Work out the finished part from the listing and answer in its coordinate system (mm). Coordinates: 2 decimals unless noted, no trailing zeros. Order: outer loops, then holes, each group sorted by start corner. A loop starts at its lowest first (then second) coordinate and runs counter-clockwise, first axis right, second up. Notation, with made-up numbers: M 5,84.5 L 33,84.5 A14 cw 33,98.5 Z; hole C 19,79.25 d8. An arc over 180 degrees is marked long. Use a Markdown table: item, result. Add a question column.
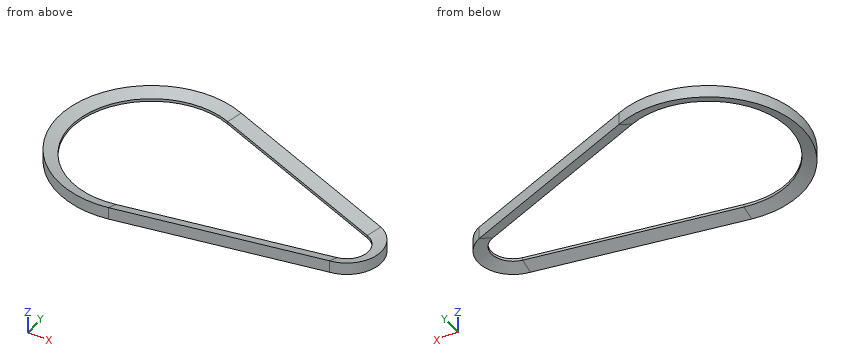
from build123d import *


with BuildPart() as part:
    # Sweep1: sweep along a path in Sketch1
    with BuildLine(Plane.XY) as sweep1_path:
        Line((18.332237974, 42.733816245), (127.408308877, -4.058365328))
        ThreePointArc((127.408308877, -4.058365328), (134.851518724, -17.062845226), (124.403812758, -27.803576593))
        Line((124.403812758, -27.803576593), (7.110625962, -45.953117396))
        ThreePointArc((7.110625962, -45.953117396), (-46.132178368, 5.837132773), (18.332237974, 42.733816245))
    # Sketch2 → Sweep1 (sweep)
    with BuildSketch(Plane(origin=(7.110625962, 0, 0), x_dir=(0, 0, -1), z_dir=(1, 0, 0))):
        Polygon((-0.770223243, -45.953117396), (0.770223243, -45.953117396), (3.5, -53.453117396), (-3.5, -53.453117396), align=None)
    sweep(path=sweep1_path.line)


solid = part.part
(1) Given P1, Ø3, axis at x = 81.5, z = 2.5, coming from the -Y side; P2, Ø1.5, axis at y = 3.5, z = 0.5, coming from the +X side; P3, Ø2, axis at x = -12.5, z = 1.5, coming from the -Y side, each flat-ended and moving along its own axis, determine where each tip first touches the part or whether it passes through.
(2) Straight lines are drawn through the part: line 1 (Y direction, x = 0, z = -0.1); line 2 (Z direction, x = 93.5, y = -40); line 3 (X direction, y = 0, z = -0.05). For each, find the intervals that lie inside material, in ascending order.
(3) A cutting plane is placed at A-A on x = 42.5. Write down the section's boundary in (y, z), plus the area to 3 significant figures.
From the geometry:
| question | item | result |
|---|---|---|
| 1 | P1 | stops at y = -42.17 |
| 1 | P2 | stops at x = 130.34 |
| 1 | P3 | stops at y = -52.68 |
| 2 | line 1 | y = -53.92 to -46.5, 46.5 to 53.92 |
| 2 | line 2 | z = -3.47 to 3.47 |
| 2 | line 3 | x = -53.92 to -46.5, 117.95 to 134.97 |
| 3 | outline | M -47.98,-3.5 L -40.48,-0.77 L -40.48,0.77 L -47.98,3.5 Z; M 32.37,-0.77 L 40.43,-3.5 L 40.43,3.5 L 32.37,0.77 Z |
| 3 | area | 66.5 mm2 |
